Verification items for this drawing (mm, ordinates from the low corner). A direction names the side the tool comes from. Round coordinates to 2 decimals unless told otherwise and drop trailing zeros. Loops run counter-clockwise (first coordinate to the right, second up) from the corner with the lowest first, then second, coordinate; pieces in that order, holes last. Notation, with made-up numbers: M -30,17.5 L -18,17.5 A17 cw -18,44.5 Z; hole C 43,69 d4. An arc over 180 degrees is marked long. Write item = value, one per line. Start each with the question number.
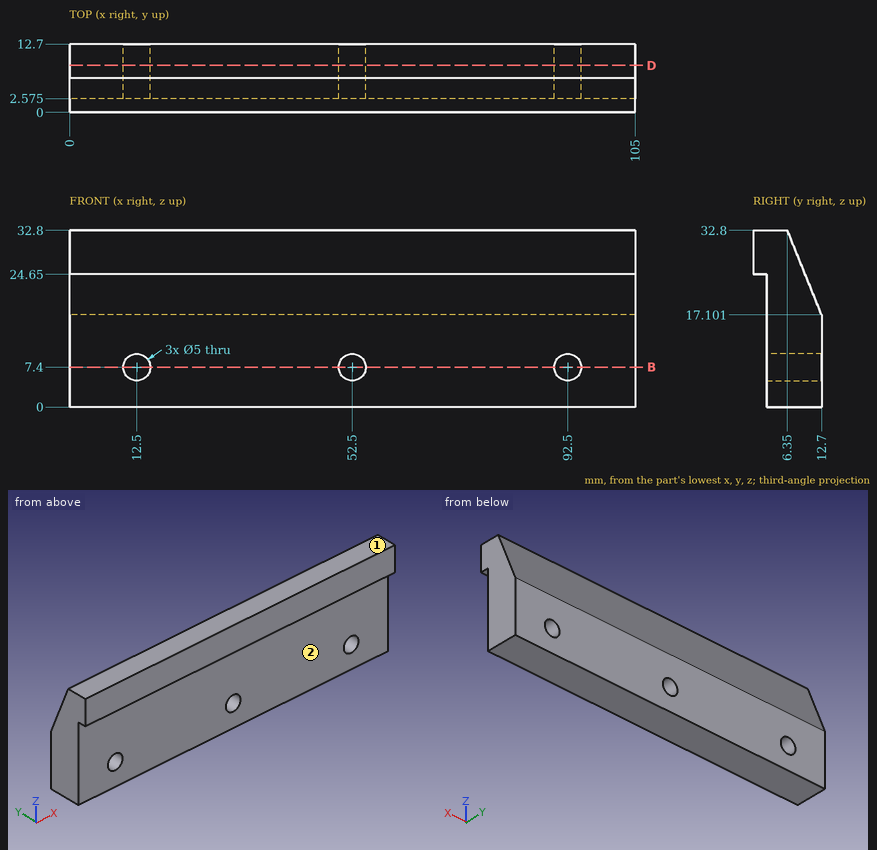
1. Section check B-B, the plane z = 7.4. Enter the section's corners in (x, y) (1 decimal), and give its area (3 significant figures).
2. Gauge pin test, flat ends, axial feed: P1, Ø1.5, axis at x = 91.5, z = 19.5, coming from the -Y side (1 decimal); P2, Ø4.5, axis at x = 12.5, z = 7.4, coming from the -Y side; P3, Ø3, axis at x = 35.5, y = 1, coming from the -Z side; P4, Ø1, axis at y = 9, z = 17.5, coming from the -X side. Record the tip position at first contact, or that the pin passes through.
3. Thickness scan on line 1 (X direction, y = 8, z = 7.4); line 2 (X direction, y = 6.75, z = 9); line 3 (Y direction, x = 43, z = 4) (1 decimal). Record the ranges inside material, lowest first.
4. Section check D-D, the plane y = 8.75. Enter the section's corners in (x, z).
5. Tool access check on the marked faces 1 and 2. Record the directions out of +Z, -Z, +X, -X, +Y, -Y that give a thin tool (end or side, any length) a straight path to the whole face; none if there is none.
Computed values:
q1.outline = M 0,2.6 L 10,2.6 L 10,12.7 L 0,12.7 Z; M 15,2.6 L 50,2.6 L 50,12.7 L 15,12.7 Z; M 55,2.6 L 90,2.6 L 90,12.7 L 55,12.7 Z; M 95,2.6 L 105,2.6 L 105,12.7 L 95,12.7 Z
q1.area = 911 mm2
q2.P1 = 2.6
q2.P2 = through
q2.P3 = 24.65
q2.P4 = 0
q3.line_1 = 0 to 10, 15 to 50, 55 to 90, 95 to 105
q3.line_2 = 0 to 10.58, 14.42 to 50.58, 54.42 to 90.58, 94.42 to 105
q3.line_3 = 2.6 to 12.7
q4.outline = M 0,0 L 105,0 L 105,26.87 L 0,26.87 Z; hole C 12.5,7.4 d5; hole C 52.5,7.4 d5; hole C 92.5,7.4 d5
q5.face_1 = +Z, +X, -X, +Y, -Y
q5.face_2 = -Z, +X, -X, -Y
